The model under review builds one solid part; all positions refer to its coordinate system, in mm. A direction names the side the tool comes from. Give positions to 0.01 mm unless a question says otherwise; leave off trailing zeros. Order: outer loops, then holes, each group sorted by start corner. A loop starts at its lowest first (then second) coordinate and runs counter-clockwise, first axis right, second up. Notation, with made-up numbers: (-29.5, 65.25) - (27.5, 65.25) arc R16 cw to (27.5, 81.25) - close; hole circle Ø6 at (30.25, 41.5). An arc over 180 degrees is marked (long way). Put each result on its own line as item: value.
```python
from build123d import *

# Parameters (mm, degrees)
SKETCH1_R                       = 25
BOSS_EXTRUDE1_DEPTH             = 10
SKETCH2_R                       = 10.037234393
BOSS_EXTRUDE2_DEPTH             = 20
SKETCH3_R                       = 6
CUT_EXTRUDE1_DEPTH              = 47.368092477
CIRPATTERN1_COUNT               = 4
M5X0_8_TAPPED_HOLE1_D           = 4.2
M5X0_8_TAPPED_HOLE1_DEPTH       = 11
M5X0_8_TAPPED_HOLE1_CSINK_D     = 5.05
M5X0_8_TAPPED_HOLE1_CSINK_ANGLE = 100
M5X0_8_TAPPED_HOLE1_TIP         = 1.2618073


with BuildPart() as part:
    # Sketch1 → Boss-Extrude1 (new body)
    with BuildSketch(Plane(origin=(0, 0, 0), x_dir=(1, 0, 0), z_dir=(0, 1, 0))):
        with Locations(Location((0, 0, 0), (0, 0, 270))):
            Circle(SKETCH1_R)
    extrude(amount=BOSS_EXTRUDE1_DEPTH)

    # Sketch2 → Boss-Extrude2 (add)
    with BuildSketch(Plane.XZ):
        with Locations(Location((0, 0, 0), (0, 0, 270))):
            Circle(SKETCH2_R)
    extrude(amount=BOSS_EXTRUDE2_DEPTH)

    # Sketch3 → Cut-Extrude1 (cut, through all)
    with BuildSketch(Plane(origin=(0, 10, 0), x_dir=(1, 0, 0), z_dir=(0, 1, 0))):
        with Locations(Location((0, 0, 0), (0, 0, 270))):
            Circle(SKETCH3_R)
    extrude(amount=-CUT_EXTRUDE1_DEPTH, mode=Mode.SUBTRACT)

    # Sketch5 → M4x0.7 Tapped Hole1 (revolve, cut)
    with BuildSketch(Plane(origin=(19, 10, 0), x_dir=(0, 0, 1), z_dir=(1, 0, 0))):
        Polygon((0, 0), (0, 9.991420021), (1.65, 9), (1.65, 0.314662362), (2.025, 0), align=None)
    m4x0_7_tapped_hole1 = revolve(axis=Axis((19, 16.35, 0), (0, -1, 0)), mode=Mode.SUBTRACT)

    # CirPattern1: M4x0.7 Tapped Hole1 ×4 about axis
    cirpattern1_axis = Axis((0, 0, 0), (0, 1, 0))
    for i in range(1, CIRPATTERN1_COUNT):
        add(m4x0_7_tapped_hole1.rotate(cirpattern1_axis, i * 360 / CIRPATTERN1_COUNT), mode=Mode.SUBTRACT)

    # M5x0.8 Tapped Hole1
    with Locations(Plane.XY.offset(10.037234393)):
        with Locations((0, -10)):
            CounterSinkHole(M5X0_8_TAPPED_HOLE1_D / 2, M5X0_8_TAPPED_HOLE1_CSINK_D / 2, depth=M5X0_8_TAPPED_HOLE1_DEPTH, counter_sink_angle=M5X0_8_TAPPED_HOLE1_CSINK_ANGLE)
            with Locations((0, 0, -(M5X0_8_TAPPED_HOLE1_DEPTH + M5X0_8_TAPPED_HOLE1_TIP / 2))):  # 118° drill point
                Cone(0, M5X0_8_TAPPED_HOLE1_D / 2, M5X0_8_TAPPED_HOLE1_TIP, mode=Mode.SUBTRACT)


solid = part.part
```
(1) For faces 4 (the flat face through (-11, 0, 0)), 5 (the cylindrical face through (0.89, 5.4, -17.61)), 6 (the cylindrical face through (2.1, -9.91, 7.62)), list the 3-axis set-ups (+Z, -Z, +X, -X, +Y, -Y) from which the entire face can be reached by the end or side of a thin tool; tool diameter is ignored.
The answers:
face 4: -Y
face 5: +Y
face 6: +Z
(2) Wall thickness on L1, parallel to X at y = 7, z = 0; L2, parallel to X at y = -4.5, z = 0; L3, parallel to Z at x = 1.5, y = 6: over which ranges is each line inside the solid? List them lowest first.
The answers:
L1: -25 to -20.65, -17.35 to -6, 6 to 17.35, 20.65 to 25
L2: -10.04 to -6, 6 to 10.04
L3: -24.95 to -19.69, -18.31 to -5.81, 5.81 to 18.31, 19.69 to 24.95
(3) Take a section at D-D, the plane x = -11. Write out the cut boundary in (y, z).
The answers:
outline: (0, -22.45) - (10, -22.45) - (10, 22.45) - (0, 22.45) - close
(4) The part is to be moulded in two halves that separate along X. For faces 1 (the conical face through (18.72, 0.18, -0.04)), 2 (the cylindrical face through (7.509, 4.93, 23.846)), 3 (the flat face through (-7, -20, 0)), say which applies: pulls with the +X half, pulls with the -X half, needs draft (parallel to the pull), parting line crosses it, or undercut.
The answers:
face 1: undercut
face 2: parting line crosses it
face 3: needs draft
(5) Take a section at C-C, the plane y = -3. Write out the cut boundary in (x, z).
The answers:
outline: circle Ø20.07 at (0, 0); hole circle Ø12 at (0, 0)
(6) Clearance check with flat-ended pins moving along their axes: pin 1 Ø6 at (y, z) = (-2.5, 13.5) entering from -X; pin 2 Ø1.5 at (y, z) = (6, 14) entering from +X; pin 3 Ø5 at (x, z) = (6, 12) entering from -Y. State where each tip first meets the part, or that it passes through.
The answers:
pin 1: x = -22.02
pin 2: x = 21.2
pin 3: y = 0
(7) Take a section at B-B, the plane z = 5. Write out the cut boundary in (x, y).
The answers:
outline: (-24.49, 0) - (-8.7, 0) - (-8.7, -20) - (-3.32, -20) - (-3.32, 10) - (-24.49, 10) - close; (3.32, -20) - (8.7, -20) - (8.7, 0) - (24.49, 0) - (24.49, 10) - (3.32, 10) - close
(8) Take a section at A-A, the plane y = 3. Write out the cut boundary in (x, z), then the cut area to 3 significant figures.
The answers:
outline: circle Ø50 at (0, 0); hole circle Ø3.3 at (-19, 0); hole circle Ø12 at (0, 0); hole circle Ø3.3 at (0, -19); hole circle Ø3.3 at (0, 19); hole circle Ø3.3 at (19, 0)
area: 1,820 mm^2
